Design review of the part built by this model. Coordinates are the model's own, in mm. A direction names the side the tool comes from. Give positions to 0.01 mm unless a question says otherwise; leave off trailing zeros. Loops run counter-clockwise (first coordinate to the right, second up) from the corner with the lowest first, then second, coordinate; pieces in that order, holes last. Notation, with made-up numbers: M -28.5,49.5 L 13.5,49.5 A29 ccw 13.5,82.5 Z; hole C -1,-36 d4. An arc over 180 degrees is marked long. Use one line per item in the form item = value. Start each with the question number.
from build123d import *

# Parameters (mm, degrees)
SKETCH1_R                = 1.2
BOSS_EXTRUDE1_DEPTH      = 1.25
SKETCH2_R                = 3
SKETCH2_R_2              = 1.2
BOSS_EXTRUDE2_DEPTH      = 0.5
BOSS_EXTRUDE2_DEPTH_BACK = 2.5


with BuildPart() as part:
    # Sketch1 → Boss-Extrude1 (new body, symmetric)
    with BuildSketch(Plane.XY):
        with BuildLine():
            Line((-6.234807428, -1.68130528), (-3.34389464, 1.5))
            Line((-3.34389464, 1.5), (3.34389464, 1.5))
            Line((3.34389464, 1.5), (6.234807428, -1.68130528))
            ThreePointArc((6.234807428, -1.68130528), (9.76630528, -1.850192572), (9.935192572, 1.68130528))
            Line((9.935192572, 1.68130528), (6.300316278, 5.68130528))
            ThreePointArc((6.300316278, 5.68130528), (5.461740431, 6.286182757), (4.450123705, 6.5))
            Line((4.450123705, 6.5), (-4.450123705, 6.5))
            ThreePointArc((-4.450123705, 6.5), (-5.461740431, 6.286182757), (-6.300316278, 5.68130528))
            Line((-6.300316278, 5.68130528), (-9.935192572, 1.68130528))
            ThreePointArc((-9.935192572, 1.68130528), (-9.76630528, -1.850192572), (-6.234807428, -1.68130528))
        make_face()
        with Locations((-8.085, 0)):
            Circle(SKETCH1_R, mode=Mode.SUBTRACT)
        with Locations((8.085, 0)):
            Circle(SKETCH1_R, mode=Mode.SUBTRACT)
    extrude(amount=BOSS_EXTRUDE1_DEPTH, both=True)

    # Sketch2 → Boss-Extrude2 (add, two sides)
    with BuildSketch(Plane.XY.offset(1.25)) as boss_extrude2_sk:
        with Locations((8.085, 0)):
            Circle(SKETCH2_R)
        with Locations((8.085, 0)):
            Circle(SKETCH2_R_2, mode=Mode.SUBTRACT)
        with Locations((-8.085, 0)):
            Circle(SKETCH2_R)
        with Locations((-8.085, 0)):
            Circle(SKETCH2_R_2, mode=Mode.SUBTRACT)
    extrude(amount=BOSS_EXTRUDE2_DEPTH)
    extrude(boss_extrude2_sk.sketch, amount=-BOSS_EXTRUDE2_DEPTH_BACK)


solid = part.part
Q1. Take a section at A-A on z = 0.2. Give the boundary of the cut face in (x, y) (3 decimals).
Q2. For faces 1 (the cylindrical face through (-5.45, 6.29, 0.02)), 2 (the flat face through (0, 1.5, 0)), list the 3-axis set-ups (+Z, -Z, +X, -X, +Y, -Y) from which the entire face can be reached by the end or side of a thin tool; tool diameter is ignored.
Q3. Take a section at C-C on x = -2.75. Give the boundary of the cut face in (y, z), plus the area to 3 significant figures.
Q4. Take a section at D-D on y = 2.25. Give the boundary of the cut face in (x, z).
Q5. Wall thickness on probe 1 along Z at (x, y) = (-6.25, 3.75); probe 2 along Y at (x, z) = (-1.75, -1.05); probe 3 along Y at (x, z) = (-7.75, 1.35): over which ranges is each line inside the solid? List them lowest first.
Q6. Clearance check with flat-ended pins moving along their axes: pin 1 Ø5.5 at (x, y) = (0, 4) entering from +Z; pin 2 Ø1.5 at (y, z) = (4, 0) entering from +X; pin 3 Ø3 at (x, y) = (8.085, 0) entering from +Z; pin 4 Ø1.5 at (x, z) = (-6, 0) entering from +Y. State where each tip first meets the part, or that it passes through.
Q7. Take a section at B-B on x = 7.75. Give the boundary of the cut face in (y, z).
Response values:
q1.outline = M -8.82,2.909 A3 ccw long -5.12,-0.454 L -3.344,1.5 L 3.344,1.5 L 5.12,-0.454 A3 ccw long 8.82,2.909 L 6.3,5.681 A2.5 ccw 4.45,6.5 L -4.45,6.5 A2.5 ccw -6.3,5.681 Z; hole C -8.085,0 d2.4; hole C 8.085,0 d2.4
q2.face_1 = +Z, -Z, -X, +Y
q2.face_2 = +Z, -Z, -Y
q3.outline = M 1.5,-1.25 L 6.5,-1.25 L 6.5,1.25 L 1.5,1.25 Z
q3.area = 12.5 mm^2
q4.outline = M -10.07,-1.25 L 10.07,-1.25 L 10.07,1.75 L 6.1,1.75 L 6.1,1.25 L -6.1,1.25 L -6.1,1.75 L -10.07,1.75 Z
q5.probe_1 = -1.25 to 1.25
q5.probe_2 = 1.5 to 6.5
q5.probe_3 = -2.98 to -1.15, 1.15 to 2.98
q6.pin_1 = 1.25
q6.pin_2 = 8.51
q6.pin_3 = 1.75
q6.pin_4 = 6.37
q7.outline = M -2.98,-1.25 L -1.15,-1.25 L -1.15,1.75 L -2.98,1.75 Z; M 1.15,-1.25 L 4.09,-1.25 L 4.09,1.25 L 2.98,1.25 L 2.98,1.75 L 1.15,1.75 Z
